Input: dimensioned drawing with shaded views. Units: mm. Origin: part minimum x, y, z. A direction names the side the tool comes from. Round coordinates to 2 decimals unless told otherwise and drop trailing zeros. Loops run counter-clockwise (first coordinate to the right, second up) from the corner with the lowest first, then second, coordinate; pieces in that order, holes last. Notation, with made-up numbers: (48, 25.5) - (90, 25.5) arc R14 ccw to (90, 51.5) - close; hole circle Ø8 at (17.25, -38). An arc over 180 degrees is marked (long way). One line per question, with ' | ' between items. Start each with the question number.
1. Cut plane B-B (y = 56). Return loops of the section in (x, z), then the cut area to 3 significant figures.
2. Pin query (flat end, axial travel): pin 1 (12 mm diameter, centred on x = 105, z = 25, fed in from -Y); pin 2 (25 mm diameter, centred on x = 72.5, z = 19.5, fed in from +Y); pin 3 (23 mm diameter, centred on x = 25, z = 25, fed in from +Y); pin 4 (8 mm diameter, centred on y = 30.5, z = 47.5, fed in from -X). Return the tip coordinate at first contact, or that it passes through.
3. Cut plane D-D (z = 25). Return loops of the section in (x, y), then the cut area to 3 significant figures.
4. Cut plane C-C (x = 25). Return loops of the section in (y, z), then the cut area to 3 significant figures.
5. Ray query, line 1 (X direction, y = 8, z = 25); line 2 (Z direction, x = 67, y = 34.5); line 3 (Y direction, x = 65, z = 45.5). Return the intervals inside material, ascending.
6. Cut plane A-A (z = 42). Return loops of the section in (x, y), then the cut area to 3 significant figures.
7. Access query for the marked faces 1, 2 and 3. Directions: +Z, -Z, +X, -X, +Y, -Y. A direction counts if a zero-diameter tool reaches every point of the face in a straight line with its end or side. Return the directions, or none.
8. Mould query, pull axis X, two halves, no side actions, for the marked faces 4, 5 and 6. Classes: pulls with the +X half, pulls with the -X half, needs draft (parallel to the pull), parting line crosses it, or undercut.
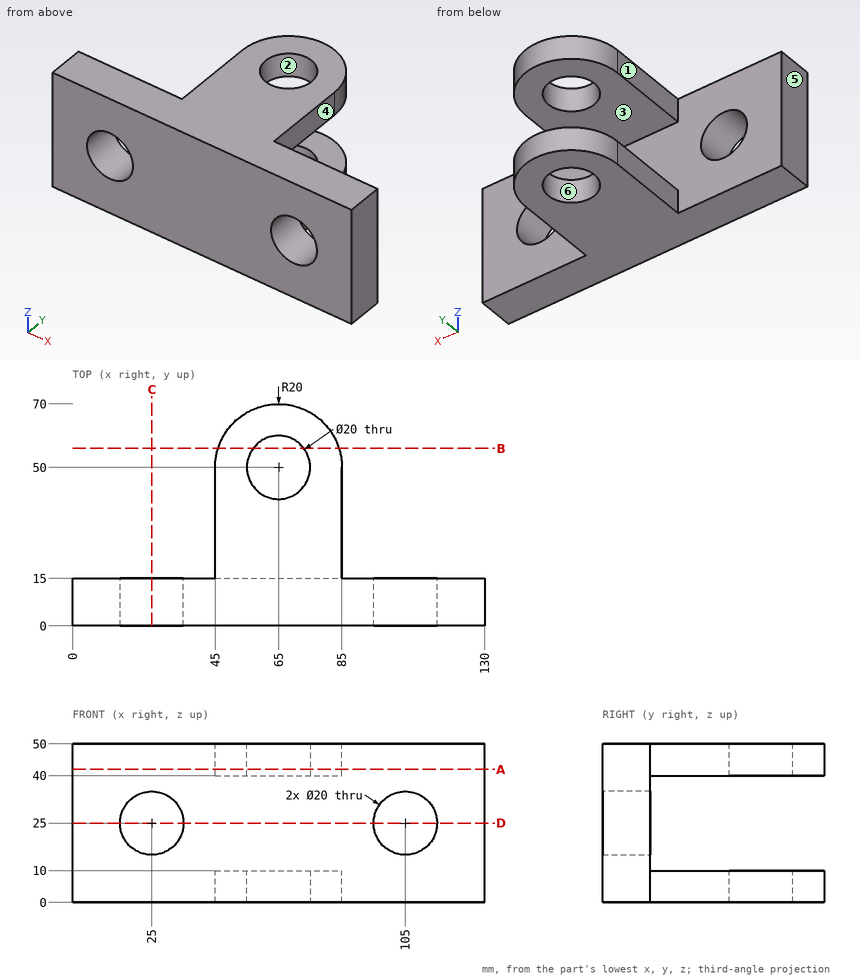
Answers follow:
1) outline: (45.92, 0) - (57, 0) - (57, 10) - (45.92, 10) - close; (45.92, 40) - (57, 40) - (57, 50) - (45.92, 50) - close; (73, 0) - (84.08, 0) - (84.08, 10) - (73, 10) - close; (73, 40) - (84.08, 40) - (84.08, 50) - (73, 50) - close | area: 443 mm2
2) pin 1: passes through | pin 2: stops at y = 70 | pin 3: stops at y = 15 | pin 4: stops at x = 45
3) outline: (0, 0) - (15, 0) - (15, 15) - (0, 15) - close; (35, 0) - (95, 0) - (95, 15) - (35, 15) - close; (115, 0) - (130, 0) - (130, 15) - (115, 15) - close | area: 1,350 mm2
4) outline: (0, 0) - (15, 0) - (15, 15) - (0, 15) - close; (0, 35) - (15, 35) - (15, 50) - (0, 50) - close | area: 450 mm2
5) line 1: x = 0 to 15, 35 to 95, 115 to 130 | line 2: z = 0 to 10, 40 to 50 | line 3: y = 0 to 40, 60 to 70
6) outline: (0, 0) - (130, 0) - (130, 15) - (85, 15) - (85, 50) arc R20 ccw to (45, 50) - (45, 15) - (0, 15) - close; hole circle Ø20 at (65, 50) | area: 3,660 mm2
7) face 1: +Z, -Z, -X, +Y | face 2: +Z, -Z | face 3: +X, -X, +Y
8) face 4: pulls with the +X half | face 5: pulls with the -X half | face 6: undercut
